from build123d import *

# Parameters (mm, degrees)
SKETCH1_W               = 32
SKETCH1_H               = 28.5
BOSS_EXTRUDE1_DEPTH     = 8
SKETCH3_R               = 11
BOSS_EXTRUDE2_DEPTH     = 28.5
SKETCH4_R               = 7.55
CUT_EXTRUDE2_DEPTH      = 26.5
SKETCH5_R               = 5
CUT_EXTRUDE3_DEPTH      = 40.398604036
SKETCH2_R               = 2
CUT_EXTRUDE1_DEPTH      = 26.594188794
CUT_EXTRUDE1_DEPTH_BACK = 26.594188794
CUT_EXTRUDE5_DEPTH      = 40.398604164


with BuildPart() as part:
    # Sketch1 → Boss-Extrude1 (new body)
    with BuildSketch(Plane(origin=(0, 0, 0), x_dir=(1, 0, 0), z_dir=(0, 1, 0))):
        Rectangle(SKETCH1_W, SKETCH1_H)
    extrude(amount=BOSS_EXTRUDE1_DEPTH)

    # Sketch3 → Boss-Extrude2 (add, through all)
    with BuildSketch(Plane.XY.offset(14.25)):
        with Locations((0, 11)):
            Circle(SKETCH3_R)
    extrude(amount=-BOSS_EXTRUDE2_DEPTH)

    # Sketch4 → Cut-Extrude2 (cut)
    with BuildSketch(Plane.XY.offset(14.25)):
        with Locations((0, 11)):
            Circle(SKETCH4_R)
    extrude(amount=-CUT_EXTRUDE2_DEPTH, mode=Mode.SUBTRACT)

    # Sketch5 → Cut-Extrude3 (cut, through all)
    with BuildSketch(Plane(origin=(0, 0, -14.25), x_dir=(-1, 0, 0), z_dir=(0, 0, -1))):
        with Locations((0, 11)):
            Circle(SKETCH5_R)
    extrude(amount=-CUT_EXTRUDE3_DEPTH, mode=Mode.SUBTRACT)

    # Sketch2 → Cut-Extrude1 (cut, two sides)
    with BuildSketch(Plane(origin=(0, 8, 0), x_dir=(1, 0, 0), z_dir=(0, 1, 0))) as cut_extrude1_sk:
        with Locations(Location((-12, 9, 0), (0, 0, 270))):
            Circle(SKETCH2_R)
        with Locations(Location((-12, -9, 0), (0, 0, 315.112762264))):
            Circle(SKETCH2_R)
        with Locations(Location((12, -9, 0), (0, 0, 270))):
            Circle(SKETCH2_R)
        with Locations(Location((12, 9, 0), (0, 0, 224.887210993))):
            Circle(SKETCH2_R)
    extrude(amount=CUT_EXTRUDE1_DEPTH, mode=Mode.SUBTRACT)
    extrude(cut_extrude1_sk.sketch, amount=-CUT_EXTRUDE1_DEPTH_BACK, mode=Mode.SUBTRACT)

    # Sketch7 → Cut-Extrude5 (cut, through all)
    with BuildSketch(Plane.XY.offset(14.25)):
        with BuildLine():
            Line((-0.435778714, 15.98097349), (-0.95871317, 21.958141679))
            ThreePointArc((-0.95871317, 21.958141679), (0, 22), (0.95871317, 21.958141679))
            Line((0.95871317, 21.958141679), (0.435778714, 15.98097349))
            ThreePointArc((0.435778714, 15.98097349), (0, 16), (-0.435778714, 15.98097349))
        make_face()
    extrude(amount=-CUT_EXTRUDE5_DEPTH, mode=Mode.SUBTRACT)


solid = part.part
The model under review builds one solid part; all positions refer to its coordinate system, in mm. A direction names the side the tool comes from. Give positions to 0.01 mm unless a question says otherwise; leave off trailing zeros. Loops run counter-clockwise (first coordinate to the right, second up) from the corner with the lowest first, then second, coordinate; pieces in that order, holes last. Notation, with made-up numbers: (83, 38) -> (131, 38) arc R31 ccw to (131, 70) -> close; hole circle Ø10 at (-5, 44.5). An arc over 180 degrees is marked (long way). Write each question's results on one line, items separated by ' | '.
1) Tool access review of faces 5 (the face through (-0.81, 20.26, 0.2)), 6 (the face through (2, 6, -12.25)), 7 (the face through (3, 6, -14.25)): name each direction out of +Z, -Z, +X, -X, +Y, -Y from which nothing blocks a thin tool from reaching the whole face with its end or side.
Conclusion:
face 5: +Z, -Z, +Y | face 6: +Z | face 7: -Z, +X, -X, +Y, -Y
2) Take a section at C-C, the plane z = 9. Give the boundary of the cut face in (x, y).
Conclusion:
outline: (-16, 0) -> (-14, 0) -> (-14, 8) -> (-16, 8) -> close; (-10, 0) -> (10, 0) -> (10, 15.58) arc R11 ccw to (0.96, 21.96) -> (0.66, 18.52) arc R7.55 cw (long way) to (-0.66, 18.52) -> (-0.96, 21.96) arc R11 ccw to (-10, 15.58) -> close; (14, 0) -> (16, 0) -> (16, 8) -> (14, 8) -> close
3) Take a section at A-A, the plane x = -12. Give the boundary of the cut face in (y, z), plus the area to 3 significant figures.
Conclusion:
outline: (0, -14.25) -> (8, -14.25) -> (8, -11) -> (0, -11) -> close; (0, -7) -> (8, -7) -> (8, 7) -> (0, 7) -> close; (0, 11) -> (8, 11) -> (8, 14.25) -> (0, 14.25) -> close | area: 164 mm^2
4) Insertion check: pin 1 Ø7.5 at (x, y) = (-1, 13) entering from +Z; pin 2 Ø1.5 at (x, z) = (-8, 10) entering from +Y; pin 3 Ø1.6 at (x, z) = (13.5, -6) entering from +Y; pin 4 Ø5 at (x, z) = (9, 0) entering from -Y. Each pin has a flat end and moves straight along its axis. Give the tip position at first contact, or say it passes through.
Conclusion:
pin 1: stops at z = -12.25 | pin 2: stops at y = 19.27 | pin 3: stops at y = 8 | pin 4: stops at y = 0
5) For line 1 along Z through (x, y) = (-12, 3.75); line 2 along X through (y, z) = (2.25, 9); line 3 along Z through (x, y) = (-13.5, 7.25), list the stretches that pass through material, from the lowest coordinate up. Write a range as from..to.
Conclusion:
line 1: z = -14.25..-11, -7..7, 11..14.25 | line 2: x = -16..-14, -10..10, 14..16 | line 3: z = -14.25..-10.32, -7.68..7.68, 10.32..14.25
6) Take a section at D-D, the plane y = 4.5. Give the boundary of the cut face in (x, z), plus the area to 3 significant figures.
Conclusion:
outline: (-16, -14.25) -> (16, -14.25) -> (16, 14.25) -> (3.84, 14.25) -> (3.84, -12.25) -> (-3.84, -12.25) -> (-3.84, 14.25) -> (-16, 14.25) -> close; hole circle Ø4 at (-12, -9); hole circle Ø4 at (-12, 9); hole circle Ø4 at (12, -9); hole circle Ø4 at (12, 9) | area: 658 mm^2
7) Take a section at B-B, the plane y = 13.25. Give the boundary of the cut face in (x, z), plus the area to 3 significant figures.
Conclusion:
outline: (-10.77, -14.25) -> (-4.47, -14.25) -> (-4.47, -12.25) -> (-7.21, -12.25) -> (-7.21, 14.25) -> (-10.77, 14.25) -> (-10.77, 10.58) arc R2 cw to (-10.77, 7.42) -> (-10.77, -7.42) arc R2 cw to (-10.77, -10.58) -> close; (4.47, -14.25) -> (10.77, -14.25) -> (10.77, -10.58) arc R2 cw to (10.77, -7.42) -> (10.77, 7.42) arc R2 cw to (10.77, 10.58) -> (10.77, 14.25) -> (7.21, 14.25) -> (7.21, -12.25) -> (4.47, -12.25) -> close | area: 207 mm^2
8) Draft analysis for pull direction X (two halves, no side actions). For faces 1 (the face through (0, 0, 0)), 2 (the face through (0.817, 20.34, 0.2)), 3 (the face through (-16, 4, 0)), 4 (the face through (16, 4, 0)), state which applies: pulls with the +X half, pulls with the -X half, needs draft (parallel to the pull), parting line crosses it, or undercut.
Conclusion:
face 1: needs draft | face 2: undercut | face 3: pulls with the -X half | face 4: pulls with the +X half
